Here's how the part is built. I have some questions about the finished solid (model axes, mm). Face numbers are marked on the shaded views. Coordinates: 2 decimals unless noted, no trailing zeros. Loops run counter-clockwise (first coordinate to the right, second up) from the corner with the lowest first, then second, coordinate; pieces in that order, holes last. Notation, with made-up numbers: M -33,45 L 2,45 A28 ccw 2,71 Z; hole C 65.5,-35 d9. An arc over 180 degrees is marked long. Use one line per item in the form item = value. Start each with the question number.
(1) Imagine slicing it at C-C, the plane x = 10. Please give me the cut outline in (y, z).
(2) Imagine slicing it at B-B, the plane z = 16. Please give me the cut outline in (x, y).
(3) Thinking about a two-plate mould opening in X: for the marked faces 1, 2, 3 and 4, which applies, +X half, -X half, draft (parallel to the pull), parting line (faces both ways), or undercut?
(4) Imagine slicing it at A-A, the plane y = 18.5. Please give me the cut outline in (x, z).
(5) Please list where these lines run through material, in increasing order: L1, parallel to X at y = 13.5, z = 63.5; L2, parallel to Z at x = -7, y = -22; L3, parallel to X at y = 19, z = 12.5.
(6) Imagine slicing it at D-D, the plane y = -23. Please give me the cut outline in (x, z).
(7) Will these pins go through, and if not, where does the flat tip stop? P1, Ø2, axis at y = 24, z = 18.5, coming from the -X side; P2, Ø0.6, axis at y = -42, z = 1, coming from the +X side; P3, Ø2, axis at y = -0.5, z = 1, coming from the -X side.
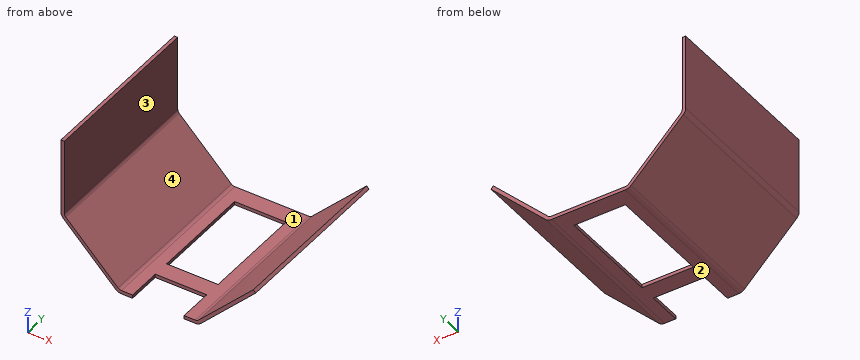
Autodesk Inventor part; units mm, degrees
ref_plane "YZ Plane" through (0, 0, 0) normal (1, 0, 0) x (0, 1, 0)
ref_plane "XZ Plane" through (0, 0, 0) normal (0, 1, 0) x (-1, 0, 0)
ref_plane "XY Plane" through (0, 0, 0) normal (0, 0, 1) x (1, 0, 0)
sketch "Sketch1" plane through (0, 0, 0) normal (0, 0, 1) x (1, 0, 0)
  line L0 (-23.5, -50) -> (23.5, -50)
  line L1 (23.5, -50) -> (23.5, 50)
  line L2 (23.5, 50) -> (-23.5, 50)
  line L3 (-23.5, 50) -> (-23.5, -50)
  line L4 (-23.5, -50) -> (23.5, 50) construction
  line L5 (23.5, -50) -> (-23.5, 50) construction
  point P0 (0, 0)
  dimension "d154" = 47
  dimension "d155" = 100
extrude "Plate3" add sketch "Sketch1" along normal blind 2
sketch "Sketch7" plane through (22.0858, 50, 1.4142) normal (0.7071068, 0, -0.7071068) x (0, 1, 0)
  line L0 (-100, 0) -> (0, 0)
  line L1 (0, 0) -> (0, 47)
  line L2 (0, 47) -> (-100, 47)
  line L3 (-100, 47) -> (-100, 0)
edge flange "Flange3" height 47 angle 45 thickness 2 bend radius 2.75 thickness toward (0.7071068, 0, -0.7071068) relief round relief width 2 relief depth 1 corner gap 2.75 corner form 0 edges at (23.5, 0, 2) (-23.5, 0, 2) wall of the first edge with corners at (22.0858, -50, 1.4142) (22.0858, 50, 1.4142) (55.3198, 50, 34.6482) (55.3198, -50, 34.6482)
bend "Bend3"
corner "Corner3"
sketch "Sketch8" plane through (0, 0, 2) normal (0, 0, 1) x (1, 0, 0)
  line L0 (15, 40) -> (-15, 40)
  line L1 (-15, 40) -> (-15, -20)
  line L2 (-15, -20) -> (15, -20)
  line L3 (15, -20) -> (15, 40)
  line L4 (15, 40) -> (-15, -20) construction
  line L5 (-15, 40) -> (15, -20) construction
  line L6 (-23.5, 50) -> (21.5325, 50)
  line L7 (-21.5325, -50) -> (21.5325, -50)
  line L8 (15, -50) -> (-15, -50)
  line L9 (-15, -50) -> (-15, -30)
  line L10 (-15, -30) -> (15, -30)
  line L11 (15, -30) -> (15, -50)
  point P0 (0, 0)
  point P1 (0, 10)
  point P2 (-15, -50)
  dimension "d166" = 30
  dimension "d168" = 10
  dimension "d182" = 10
  dimension "d183" = 20
extrude "Cut1" cut sketch "Sketch8" against normal blind 2
sketch "Sketch9" plane through (-54.734, -50, 33.234) normal (-1, 0, 0) x (0, -1, 0)
  line L0 (-100, 0) -> (0, 0)
  line L1 (0, 0) -> (0, 46)
  line L2 (0, 46) -> (-100, 46)
  line L3 (-100, 46) -> (-100, 0)
edge flange "Flange4" height 46 angle 45 thickness 2 bend radius 2.75 thickness toward (-1, 0, 0) relief round relief width 2 relief depth 1 edges at (-55.3198, 0, 34.6482) wall of the first edge with corners at (-54.734, 50, 33.234) (-54.734, -50, 33.234) (-54.734, -50, 79.234) (-54.734, 50, 79.234)
bend "Bend4"
corner "Corner4"
properties part number "MNT-CDF-503  main tube 1" material "Stainless Steel"
Answer:
q1.outline = M -30,0 L -20,0 L -20,2 L -30,2 Z; M 40,0 L 50,0 L 50,2 L 40,2 Z
q2.outline = M -39.5,-50 L -36.67,-50 L -36.67,50 L -39.5,50 Z; M 36.67,-50 L 39.5,-50 L 39.5,50 L 36.67,50 Z
q3.face_1 = undercut
q3.face_2 = draft
q3.face_3 = +X half
q3.face_4 = undercut
q4.outline = M -56.73,35.2 A4.75 ccw -55.34,31.84 L -24.89,1.39 A4.75 ccw -21.53,0 L -15,0 L -15,2 L -21.53,2 A2.75 cw -23.48,2.81 L -53.93,33.26 A2.75 cw -54.73,35.2 L -54.73,79.23 L -56.73,79.23 Z; M 15,0 L 21.53,0 A4.75 ccw 24.89,1.39 L 56.73,33.23 L 55.32,34.65 L 23.48,2.81 A2.75 cw 21.53,2 L 15,2 Z
q5.L1 = -56.73 to -54.73
q5.L2 = 0 to 2
q5.L3 = -36 to -33.17, 33.17 to 36
q6.outline = M -56.73,35.2 A4.75 ccw -55.34,31.84 L -24.89,1.39 A4.75 ccw -21.53,0 L 21.53,0 A4.75 ccw 24.89,1.39 L 56.73,33.23 L 55.32,34.65 L 23.48,2.81 A2.75 cw 21.53,2 L -21.53,2 A2.75 cw -23.48,2.81 L -53.93,33.26 A2.75 cw -54.73,35.2 L -54.73,79.23 L -56.73,79.23 Z
q7.P1 = -43
q7.P2 = 24.8
q7.P3 = -25.5
